The model under review builds one solid part; all positions refer to its coordinate system, in mm. A direction names the side the tool comes from. Coordinates: 2 decimals unless noted, no trailing zeros. Order: outer loops, then holes, each group sorted by start corner. A loop starts at its lowest first (then second) coordinate and runs counter-clockwise, first axis right, second up. Notation, with made-up numbers: M 87,5 L 145,5 A14 cw 145,23 Z; hole C -16,-11 d4. An arc over 180 degrees is marked long. Write each question's results on one line, items separated by ' | '.
from build123d import *

# Parameters (mm, degrees)
F0_W     = 138.3417099714
F0_H     = 101.5456728637
F1_DEPTH = 76.2
F2_W     = 76.2257091701
F2_H     = 63.8742726296
F3_DEPTH = 101.6
F5_DEPTH = 254
F7_DEPTH = 101.6


with BuildPart() as f1:
    # F0 (on Front) → F1 (new body)
    with BuildSketch(Plane.XZ):
        with Locations((0.7131025195, -0.7131006569)):
            Rectangle(F0_W, F0_H)
    extrude(amount=F1_DEPTH)

    # F2 (on face) → F3 (cut)
    with BuildSketch(Plane.XZ.offset(76.2)):
        with Locations((1.7188172787, 2.7152718976)):
            Rectangle(F2_W, F2_H)
    extrude(amount=-F3_DEPTH, mode=Mode.SUBTRACT)

    # F4 (on face) → F5 (join)
    with BuildSketch(Plane.YZ.offset(69.8839575052)):
        with BuildLine():
            Line((0, 50.059735775), (-50.4431385903, 50.059735775))
            ThreePointArc((-50.4431385903, 50.059735775), (-47.9958991329, 2.1220411863), (0, 2.7586021562))
            Line((0, 2.7586021562), (0, 50.059735775))
        make_face()
    extrude(amount=F5_DEPTH)

    # F6 (on face) → F7 (cut)
    with BuildSketch(Plane.XZ.offset(76.2)):
        Polygon((31.9183138803, 50.059735775), (59.1486387648, 50.059735775), (57.3735188693, 53.4748122682), (34.7362639383, 54.4770613606), align=None)
        Polygon((55.6375725195, 14.2659365838), (67.8241731599, 33.3692498798), (59.1486387648, 50.059735775), (31.9183138803, 50.059735775), (22.5496632978, 35.3737480645), (22.9246079661, 34.6524082124), (39.8316718638, 34.6524082124), (39.8316718638, 14.9657321038), align=None)
    extrude(amount=-F7_DEPTH, mode=Mode.SUBTRACT)


solid = f1.part
1) For pin 1 (10 mm diameter, centred on x = 179, y = -11, fed in from -Z); pin 2 (1 mm diameter, centred on y = -43, z = -4, fed in from +X); pin 3 (5 mm diameter, centred on x = 185.5, z = -12, fed in from -Y); pin 4 (8 mm diameter, centred on x = 195.5, z = 33, fed in from -Y), all flat-tipped, find the tip position at first contact; note any pin that passes through.
Solutions:
pin 1: z = -6.22 | pin 2: x = 69.88 | pin 3: through | pin 4: y = -58.89
2) Take a section at A-A on x = 6. State the section outline as (y, z) points.
Solutions:
outline: M -76.2,-51.49 L 0,-51.49 L 0,-29.22 L -76.2,-29.22 Z; M -76.2,34.65 L 0,34.65 L 0,50.06 L -76.2,50.06 Z
3) Take a section at B-B on z = 6.5. State the section outline as (x, y) points, plus the area to 3 significant figures.
Solutions:
outline: M -68.46,-76.2 L -36.39,-76.2 L -36.39,0 L -68.46,0 Z; M 39.83,-76.2 L 69.88,-76.2 L 69.88,-51.93 L 323.88,-51.93 L 323.88,0 L 39.83,0 Z | area: 17,900 mm2
4) To check wall thickness, follow line 1 along Z through (x, y) = (-28, -8); line 2 along X through (y, z) = (-70.5, -1.5); line 3 along X through (y, z) = (-8.5, 1). State the ranges of each line that lie inside material, in increasing order.
Solutions:
line 1: -51.49 to -29.22, 34.65 to 50.06 | line 2: -68.46 to -36.39, 39.83 to 69.88 | line 3: -68.46 to -36.39, 39.83 to 323.88
5) The part is to be moulded in two halves that separate along X. For faces 5 (the flat face through (1, -39, -29.222)), 6 (the flat face through (69.884, -46, -13)), 7 (the flat face through (27.3, -38.63, 42.82)), 8 (the flat face through (-19, -38, 50.06)), say which applies: pulls with the +X half, pulls with the -X half, needs draft (parallel to the pull), parting line crosses it, or undercut.
Solutions:
face 5: undercut | face 6: pulls with the +X half | face 7: undercut | face 8: needs draft
6) Take a section at C-C on y = -55.5. State the section outline as (x, z) points, plus the area to 3 significant figures.
Solutions:
outline: M -68.46,-51.49 L 69.88,-51.49 L 69.88,12.34 L 323.88,12.34 L 323.88,42.38 L 69.88,42.38 L 69.88,50.06 L 59.15,50.06 L 67.82,33.37 L 55.64,14.27 L 39.83,14.97 L 39.83,-29.22 L -36.39,-29.22 L -36.39,34.65 L 22.92,34.65 L 22.55,35.37 L 31.92,50.06 L -68.46,50.06 Z | area: 15,800 mm2
7) Take a section at D-D on z = 29.5. State the section outline as (x, y) points, plus the area to 3 significant figures.
Solutions:
outline: M -68.46,-76.2 L -36.39,-76.2 L -36.39,0 L -68.46,0 Z; M 65.36,-76.2 L 69.88,-76.2 L 69.88,-58.86 L 323.88,-58.86 L 323.88,0 L 65.36,0 Z | area: 17,700 mm2
8) For faces 1 (the cylindrical face through (195.106, -48.532, 2.636)), 2 (the flat face through (125, 0, 10)), 3 (the flat face through (39.832, -39, -7)), 4 (the flat face through (-7, -39, 34.652)), list the 3-axis set-ups (+Z, -Z, +X, -X, +Y, -Y) from which the entire face can be reached by the end or side of a thin tool; tool diameter is ignored.
Solutions:
face 1: +X | face 2: +Z, -Z, +X, -X, +Y | face 3: +Z, +Y, -Y | face 4: +Y, -Y
